from build123d import *

# Parameters (mm, degrees)
F0_R     = 17.7
F1_DEPTH = 6
F2_R     = 15.75
F3_DEPTH = 3
F4_R     = 15.25
F5_DEPTH = 2
F6_R     = 15.25
F7_DEPTH = 1


# Not quite as in the source:
# - a fillet or chamfer that OpenCascade refuses, or shapes differently, is made with other operations: its cross-section is extruded or revolved along the edge and cut away or added


with BuildPart() as f1:
    # F0 (on Top) → F1 (new body)
    with BuildSketch(Plane.XY):
        Circle(F0_R)
    extrude(amount=F1_DEPTH)

    # F2 (on face) → F3 (cut)
    with BuildSketch(Plane(origin=(0, 0, 0), x_dir=(1, 0, 0), z_dir=(0, 0, -1))):
        Circle(F2_R)
    extrude(amount=-F3_DEPTH, mode=Mode.SUBTRACT)

    # F4 (on face) → F5 (cut)
    with BuildSketch(Plane(origin=(0, 0, 3), x_dir=(1, 0, 0), z_dir=(0, 0, -1))):
        Circle(F4_R)
    extrude(amount=-F5_DEPTH, mode=Mode.SUBTRACT)

    # F6 (on face) → F7 (cut)
    with BuildSketch(Plane.XY.offset(6)):
        Circle(F6_R)
    extrude(amount=-F7_DEPTH, mode=Mode.SUBTRACT)

    # F8: fillet of radius 8 on 1 edges, made by hand

    # F8_s1 → F8_t2 (revolve, cut)
    with BuildSketch(Plane.XZ):
        with BuildLine():
            ThreePointArc((17.7, 0.2382728284), (17.0620649277, 3.3687679969), (15.25, 6))
            Line((15.25, 6), (15.361, 6.1152345434))
            ThreePointArc((15.361, 6.1152345434), (16.475, 6.16), (17.7, 6.16))
            Line((17.7, 6.16), (17.86, 6))
            Line((17.86, 6), (17.86, 0.2382728284))
            Line((17.86, 0.2382728284), (17.7, 0.2382728284))
        make_face()
    revolve(axis=Axis((0, 0, 6), (0, 0, 1)), mode=Mode.SUBTRACT)


solid = f1.part
Here's how the part is built. I have some questions about the finished solid (model axes, mm). Coordinates: 2 decimals unless noted, no trailing zeros. Order: outer loops, then holes, each group sorted by start corner. A loop starts at its lowest first (then second) coordinate and runs counter-clockwise, first axis right, second up.
Item 1: I need wall thicknesses on line 1 (Y direction, x = -5.5, z = 0.4); line 2 (Y direction, x = 1, z = 4.5); line 3 (X direction, y = -14.5, z = 0.85). Which ranges of each line are inside material? Lowest first, please.
Result sheet:
line 1: y = -16.82 to -14.76, 14.76 to 16.82
line 2: y = -16.44 to -15.22, 15.22 to 16.44
line 3: x = -10.11 to -6.15, 6.15 to 10.11
Item 2: If we section it at A-A on y = 0: List the corners of the cut face in (x, z) for me, plus the area to 3 significant figures.
Result sheet:
outline: (-17.7, 0) - (-15.75, 0) - (-15.75, 3) - (-15.25, 3) - (-15.25, 6) arc R8 ccw to (-17.7, 0.24) - close; (15.25, 3) - (15.75, 3) - (15.75, 0) - (17.7, 0) - (17.7, 0.24) arc R8 ccw to (15.25, 6) - close
area: 17.7 mm2
Item 3: If we mould it in two halves opening along Y, with no side actions, what happens to faces 1 (the face through (-2.05, -15.616, 1.479)), 2 (the face through (-16, -1, 0))? For each: +Y half, -Y half, draft (parallel to the pull), parting line (faces both ways), or undercut.
Result sheet:
face 1: undercut
face 2: draft
Item 4: If we section it at D-D on z = 2.4: List the corners of the cut face in (x, y) for me, plus the area to 3 significant figures.
Result sheet:
outline: circle Ø34.8 at (0, 0); hole circle Ø31.5 at (0, 0)
area: 172 mm2
Item 5: If we section it at C-C on z = 5.05: List the corners of the cut face in (x, y) for me, plus the area to 3 significant figures.
Result sheet:
outline: circle Ø32.18 at (0, 0); hole circle Ø30.5 at (0, 0)
area: 82.8 mm2
Item 6: For P1, Ø19, axis at x = 0, y = 0, coming from the -Z side; P2, Ø2, axis at y = 10.5, z = 1, coming from the +X side; P3, Ø3, axis at y = 13, z = 5, coming from the -X side; P4, Ø3, axis at y = 8.5, z = 5, coming from the -X side, each with a flat end and sliding along its axis, tell me the tip position at first contact or that it passes through.
Result sheet:
P1: passes through
P2: stops at x = 14.9
P3: stops at x = -11.83
P4: stops at x = -15.06
